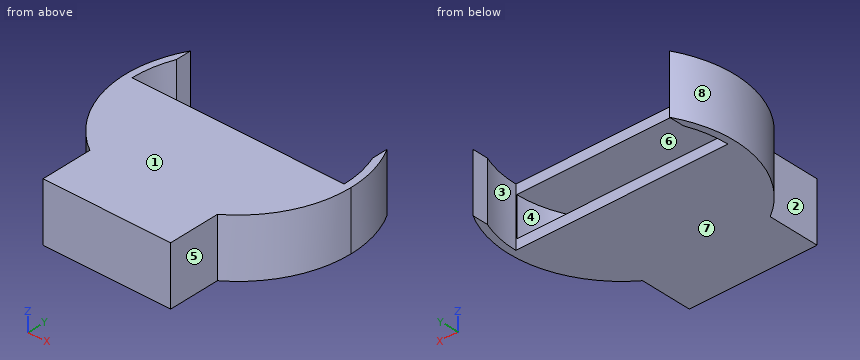
```python
from build123d import *

# Parameters (mm, degrees)
F1_DEPTH = 3
F2_R     = 10.7
F3_DEPTH = 2
F5_DEPTH = 6.001


with BuildPart() as f1:
    # F0 (on Top) → F1 (new body, symmetric)
    with BuildSketch(Plane.XY):
        with BuildLine():
            ThreePointArc((6.5, -9.486833), (10.173495, -5.361903), (11.5, 0))
            ThreePointArc((11.5, 0), (-5.361903, 10.173495), (-6.5, -9.486833))
            ThreePointArc((-6.5, -9.486833), (0, -11.5), (6.5, -9.486833))
        make_face()
        with BuildLine():
            ThreePointArc((6.5, -9.486833), (0, -11.5), (-6.5, -9.486833))
            Line((-6.5, -9.486833), (-6.5, -14.736833))
            Line((-6.5, -14.736833), (6.5, -14.736833))
            Line((6.5, -14.736833), (6.5, -9.486833))
        make_face()
    extrude(amount=F1_DEPTH, both=True)

    # F2 (on Top) → F3 (cut, symmetric)
    with BuildSketch(Plane.XY):
        Circle(F2_R)
    extrude(amount=F3_DEPTH, both=True, mode=Mode.SUBTRACT)

    # F4 (on face) → F5 (cut, through all)
    with BuildSketch(Plane.XY.offset(3)):
        with BuildLine():
            Line((-10.8, 0), (10.8, 0))
            ThreePointArc((10.8, 0), (10.598113, 2.078461), (10, 4.079216))
            Line((10, 4.079216), (10, 14.079216))
            Line((10, 14.079216), (-10, 14.079216))
            Line((-10, 14.079216), (-10, 4.079216))
            ThreePointArc((-10, 4.079216), (-10.598113, 2.078461), (-10.8, 0))
        make_face()
    extrude(amount=-F5_DEPTH, mode=Mode.SUBTRACT)


solid = f1.part
```
Check sheet for the modelled part. Datum: model origin and axes. Units: mm. Face numbers are marked on the shaded views. A direction names the side the tool comes from. Coordinates: 2 decimals unless noted, no trailing zeros. Loops run counter-clockwise (first coordinate to the right, second up) from the corner with the lowest first, then second, coordinate; pieces in that order, holes last.
1) Access from +Z, -Z, +X, -X, +Y, -Y to the whole of each face (thin tool, end or side, straight path). Record for the marked faces 1, 2, 3 and 4.
2) Release check for a two-part mould opening along X. For the marked faces 5, 6, 7 and 8 record: released by +X, released by -X, zero draft, split by the parting line, or undercut.
3) Sectioned sample at D-D (y = -8.5). Record the boundary of the cut face in (x, z).
4) Sectioned sample at B-B (x = 0). Record the boundary of the cut face in (y, z), and give its area (3 significant figures).
5) Material ranges on probe 1 along Z at (x, y) = (-0.5, -5.25); probe 2 along Y at (x, z) = (4.75, 2.6); probe 3 along X at (y, z) = (4.5, 1.9), recorded low to high.
6) Sectioned sample at A-A (y = 0.75). Record the boundary of the cut face in (x, z).
7) Sectioned sample at C-C (z = 0.7). Record the boundary of the cut face in (x, y), and give its area (3 significant figures).
8) Gauge pin test, flat ends, axial feed: pin 1 (1.8 mm diameter, centred on y = 5, z = 1, fed in from -X); pin 2 (2 mm diameter, centred on y = -2.5, z = -2, fed in from +X); pin 3 (1.3 mm diameter, centred on y = 4.5, z = -1.5, fed in from +X); pin 4 (2 mm diameter, centred on y = -0.5, z = -0.5, fed in from -X). Record the tip position at first contact, or that the pin passes through.
Check sheet entries:
1. face 1: +Z, +X, -X, +Y, -Y
1. face 2: +Z, -Z, -X, -Y
1. face 3: +Z, -Z
1. face 4: none
2. face 5: released by +X
2. face 6: undercut
2. face 7: zero draft
2. face 8: released by -X
3. outline: (-7.75, -3) - (7.75, -3) - (7.75, 3) - (-7.75, 3) - close; hole (-6.5, -2) - (6.5, -2) - (6.5, 2) - (-6.5, 2) - close
4. outline: (-14.74, -3) - (0, -3) - (0, -2) - (-10.7, -2) - (-10.7, 2) - (0, 2) - (0, 3) - (-14.74, 3) - close
4. area: 45.6 mm2
5. probe 1: z = -3 to -2, 2 to 3
5. probe 2: y = -14.74 to 0
5. probe 3: x = -10.58 to -10, 10 to 10.58
6. outline: (-11.48, -3) - (-10.77, -3) - (-10.77, 3) - (-11.48, 3) - close; (10.77, -3) - (11.48, -3) - (11.48, 3) - (10.77, 3) - close
7. outline: (-10.8, 0) arc R10.8 cw to (-10, 4.08) - (-10, 5.68) arc R11.5 ccw to (-6.5, -9.49) - (-6.5, -14.74) - (6.5, -14.74) - (6.5, -9.49) arc R11.5 ccw to (11.5, 0) arc R11.5 ccw to (10, 5.68) - (10, 4.08) arc R10.8 cw to (10.8, 0) - (10.7, 0) arc R10.7 cw to (-10.7, 0) - close
7. area: 85.5 mm2
8. pin 1: stops at x = -10.74
8. pin 2: stops at x = 11.4
8. pin 3: stops at x = 10.84
8. pin 4: stops at x = -11.5
